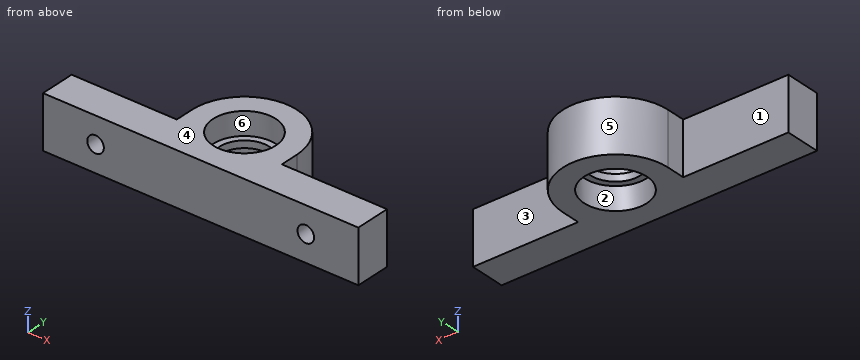
Autodesk Inventor part; units mm, degrees
ref_plane "YZ Plane" through (0, 0, 0) normal (1, 0, 0) x (0, 1, 0)
ref_plane "XZ Plane" through (0, 0, 0) normal (0, 1, 0) x (-1, 0, 0)
ref_plane "XY Plane" through (0, 0, 0) normal (0, 0, 1) x (1, 0, 0)
sketch "Sketch1" plane through (0, 0, 0) normal (0, 0, 1) x (1, 0, 0)
  line L0 (0, 0) -> (76.2, 0)
  line L1 (50.8, 8.5) -> (50.8, 13)
  line L2 (25.4, 8.5) -> (25.4, 13)
  arc A0 (50.8, 13) -> (25.4, 13) centre (38.1, 13) ccw
  line L3 (0, 8.5) -> (25.4, 8.5)
  line L4 (76.2, 8.5) -> (50.8, 8.5)
  line L5 (76.2, 8.5) -> (76.2, 0)
  line L6 (0, 8.5) -> (0, 0)
  dimension "d0" = 76.2
  dimension "d4" = 25.4
  dimension "d18" = 13
  dimension "d20" = 25.4
  dimension "d21" = 8.5
  dimension "d22" = 8.5
  dimension "d23" = 12.7
  dimension "d24" = 25.4
  dimension "d25" = 12.7
extrude "BearingBlock" add sketch "Sketch1" along normal blind 12.7
sketch "Sketch2" plane through (0, 0, 12.7) normal (0, 0, 1) x (1, 0, 0)
  arc A0 (50.8, 13) -> (25.4, 13) centre (38.1, 13) ccw
  line L0 (0, 0) -> (76.2, 0)
  circle A1 centre (38.1, 13) radius 7.575
  point P0 (38.1, 25.7)
  dimension "d8" = 15.15
  dimension "d26" = 13
extrude "BearingMount" cut sketch "Sketch2" against normal blind 5.5
sketch "Sketch4" plane through (0, 0, 0) normal (0, 0, -1) x (-1, 0, 0)
  circle A0 centre (-38.1, 13) radius 7.575
  circle A1 centre (-38.1, 13) radius 7.575
  line L0 (0, 0) -> (-76.2, 0)
  dimension "d27" = 15.15
  dimension "d28" = 13
extrude "BearingMount2" cut sketch "Sketch4" against normal blind 5.5
sketch "Sketch3" plane through (0, 0, 0) normal (0, -1, 0) x (1, 0, 0)
  line L0 (0, 0) -> (0, 12.7)
  line L1 (-76.2, 6.35) -> (76.2, 6.35) construction
  line L2 (76.2, 0) -> (76.2, 12.7)
  circle A0 centre (12.7, 6.35) radius 2
  circle A1 centre (63.5, 6.35) radius 2
  point P0 (0, 6.35)
  dimension "d11" = 12.7
  dimension "d12" = 12.7
  dimension "d13" = 4
  dimension "d14" = 4
  dimension "d15" = 50.8
extrude "HeatSetInsert" cut sketch "Sketch3" against normal blind 7
sketch "Sketch5" plane through (38.1, 13, 5.5) normal (0, 0, -1) x (-1, 0, 0)
  circle A0 centre (0, 0) radius 7.575
  circle A1 centre (0, 0) radius 6
  line L0 (38.1, -13) -> (-38.1, -13)
  dimension "d32" = 12
  dimension "d33" = 13
extrude "Extrusion5" cut sketch "Sketch5" against normal through all contours A1
equation "\"d18\" = motor_centerline_height"
equation "\"d13\" = m3_heat_set_insert"
equation "\"d14\" = m3_heat_set_insert"
equation "\"m3_heat_set_insert\" = 4"
equation "\"m3_clearance\" = 3.4"
equation "\"m3_heat_set_depth\" = 7"
equation "\"robot_diameter\" = 354"
equation "\"hardboard_thickness\" = 5"
equation "\"motor_centerline_height\" = 13"
properties part number "wheel_bearing_no_flange"
For this review, take the finished solid that the model builds, in its own axes (mm). Face numbers are marked on the shaded views. A direction names the side the tool comes from. Round coordinates to 2 decimals unless told otherwise and drop trailing zeros. Order: outer loops, then holes, each group sorted by start corner. A loop starts at its lowest first (then second) coordinate and runs counter-clockwise, first axis right, second up. Notation, with made-up numbers: (5, -18.75) -> (50, -18.75) arc R19 cw to (50, -6.75) -> close; hole circle Ø1 at (42.25, 75.25). An arc over 180 degrees is marked (long way). Use a Markdown table: item, result.
Item 1: Take a section at B-B (y = 11.25). State the section outline as (x, z) points.
Resolved:
| item | result |
|---|---|
| outline | (25.4, 0) -> (30.73, 0) -> (30.73, 5.5) -> (32.36, 5.5) -> (32.36, 7.2) -> (30.73, 7.2) -> (30.73, 12.7) -> (25.4, 12.7) -> close; (43.84, 5.5) -> (45.47, 5.5) -> (45.47, 0) -> (50.8, 0) -> (50.8, 12.7) -> (45.47, 12.7) -> (45.47, 7.2) -> (43.84, 7.2) -> close |
Item 2: For pin 1 (5 mm diameter, centred on x = 54, z = 7.5, fed in from +Y); pin 2 (3 mm diameter, centred on y = 21.5, z = 4, fed in from +X); pin 3 (4 mm diameter, centred on y = 3, z = 9, fed in from -X); pin 4 (1.2 mm diameter, centred on x = 12, z = 7.5, fed in from -Y), all flat-tipped, find the tip position at first contact; note any pin that passes through.
Resolved:
| item | result |
|---|---|
| pin 1 | stops at y = 8.5 |
| pin 2 | stops at x = 48.7 |
| pin 3 | stops at x = 0 |
| pin 4 | stops at y = 7 |
Item 3: For line 1 along Z through (x, y) = (63.5, 3.25); line 2 along Y through (x, z) = (38.1, 6.05); line 3 along Y through (x, z) = (65, 10.25), list the stretches that pass through material, from the lowest coordinate up. Write a range as [from, to].
Resolved:
| item | result |
|---|---|
| line 1 | z = [0, 4.35], [8.35, 12.7] |
| line 2 | y = [0, 7], [19, 25.7] |
| line 3 | y = [0, 8.5] |
Item 4: Take a section at A-A (z = 6.35). State the section outline as (x, y) points.
Resolved:
| item | result |
|---|---|
| outline | (0, 0) -> (10.7, 0) -> (10.7, 7) -> (14.7, 7) -> (14.7, 0) -> (61.5, 0) -> (61.5, 7) -> (65.5, 7) -> (65.5, 0) -> (76.2, 0) -> (76.2, 8.5) -> (50.8, 8.5) -> (50.8, 13) arc R12.7 ccw to (25.4, 13) -> (25.4, 8.5) -> (0, 8.5) -> close; hole circle Ø12 at (38.1, 13) |
Item 5: Take a section at D-D (z = 1). State the section outline as (x, y) points (3 decimals).
Resolved:
| item | result |
|---|---|
| outline | (0, 0) -> (76.2, 0) -> (76.2, 8.5) -> (50.8, 8.5) -> (50.8, 13) arc R12.7 ccw to (25.4, 13) -> (25.4, 8.5) -> (0, 8.5) -> close; hole circle Ø15.15 at (38.1, 13) |
Item 6: Draft analysis for pull direction Y (two halves, no side actions). For the marked faces 4, 5 and 6, state which applies: +Y half, -Y half, draft (parallel to the pull), parting line (faces both ways), or undercut.
Resolved:
| item | result |
|---|---|
| face 4 | draft |
| face 5 | +Y half |
| face 6 | undercut |
Item 7: Machinability: for the marked faces 1, 2 and 3, which of the approach directions +Z, -Z, +X, -X, +Y, -Y give a long, thin tool a straight path to every point of the face, cutting with its end or side? Answer none if there is none.
Resolved:
| item | result |
|---|---|
| face 1 | +Z, -Z, -X, +Y |
| face 2 | -Z |
| face 3 | +Z, -Z, +X, +Y |
Item 8: Take a section at C-C (x = 12.7). State the section outline as (y, z) points.
Resolved:
| item | result |
|---|---|
| outline | (0, 0) -> (8.5, 0) -> (8.5, 12.7) -> (0, 12.7) -> (0, 8.35) -> (7, 8.35) -> (7, 4.35) -> (0, 4.35) -> close |
